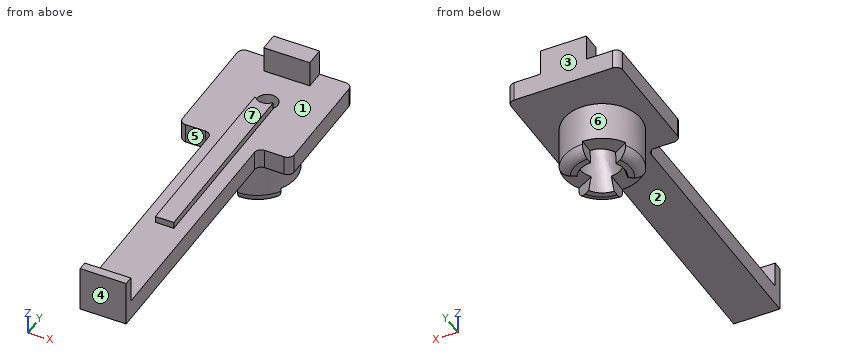
from build123d import *

# Parameters (mm, degrees)
SKETCH1_W           = 7
SKETCH1_H           = 56.5
BOSS_EXTRUDE1_DEPTH = 3
SKETCH2_W           = 2.8
SKETCH2_H           = 29
BOSS_EXTRUDE2_DEPTH = 1
SKETCH3_W           = 7
SKETCH3_H           = 2.85
SKETCH3_H_2         = 1.35
BOSS_EXTRUDE3_DEPTH = 4
SKETCH4_W           = 3
SKETCH4_H           = 18
BOSS_EXTRUDE4_DEPTH = 5
SKETCH5_W           = 3
SKETCH5_H           = 18
BOSS_EXTRUDE5_DEPTH = 5
SKETCH9_R           = 5.85
BOSS_EXTRUDE7_DEPTH = 8
FILLET1_R           = 1.5
FILLET2_R           = 1
SKETCH11_R          = 3.436863838
SKETCH7_R           = 1.6
CUT_EXTRUDE5_START  = -2
CUT_EXTRUDE5_DEPTH  = 2
SKETCH14_R          = 1.6
CUT_EXTRUDE6_DEPTH  = 3


with BuildPart() as part:
    # Sketch1 → Boss-Extrude1 (new body)
    with BuildSketch(Plane.XY):
        with Locations((0, 9.795104227)):
            Rectangle(SKETCH1_W, SKETCH1_H)
    extrude(amount=BOSS_EXTRUDE1_DEPTH)

    # Sketch2 → Boss-Extrude2 (add)
    with BuildSketch(Plane.XY.offset(3)):
        with Locations((0, 13.995104227)):
            Rectangle(SKETCH2_W, SKETCH2_H)
    extrude(amount=BOSS_EXTRUDE2_DEPTH)

    # Sketch3 → Boss-Extrude3 (add)
    with BuildSketch(Plane.XY.offset(3)):
        with Locations((0, 36.620104227)):
            Rectangle(SKETCH3_W, SKETCH3_H)
        with Locations((0, -17.779895773)):
            Rectangle(SKETCH3_W, SKETCH3_H_2)
    extrude(amount=BOSS_EXTRUDE3_DEPTH)

    # Sketch4 → Boss-Extrude4 (add)
    with BuildSketch(Plane.ZY.offset(3.5)):
        with Locations((1.5, 29.045104227)):
            Rectangle(SKETCH4_W, SKETCH4_H)
    extrude(amount=BOSS_EXTRUDE4_DEPTH)

    # Sketch5 → Boss-Extrude5 (add)
    with BuildSketch(Plane(origin=(3.5, 0, 0), x_dir=(0, 0, -1), z_dir=(1, 0, 0))):
        with Locations((-1.5, 29.045104227)):
            Rectangle(SKETCH5_W, SKETCH5_H)
    extrude(amount=BOSS_EXTRUDE5_DEPTH)

    # Sketch9 → Boss-Extrude7 (add)
    with BuildSketch(Plane(origin=(0, 0, 0), x_dir=(-1, 0, 0), z_dir=(0, 0, -1))):
        with Locations(Location((0, 26.670104227, 0), (0, 0, 180))):
            Circle(SKETCH9_R)
    extrude(amount=BOSS_EXTRUDE7_DEPTH)

    # Fillet1
    fillet1_edges = [part.edges().sort_by_distance(p)[0] for p in [
        (-5.85, 26.670104227, -8),
    ]]
    fillet(fillet1_edges, radius=FILLET1_R)

    # Fillet2
    fillet2_edges = [part.edges().sort_by_distance(p)[0] for p in [
        (-3.5, 20.045104227, 1.5),
        (-8.5, 20.045104227, 1.5),
        (-8.5, 38.045104227, 1.5),
        (3.5, 20.045104227, 1.5),
        (8.5, 38.045104227, 1.5),
        (8.5, 20.045104227, 1.5),
    ]]
    fillet(fillet2_edges, radius=FILLET2_R)

    # Sketch11 → Cut-Loft6 section 0
    with BuildSketch(Plane(origin=(0, 0, -8), x_dir=(-1, 0, 0), z_dir=(0, 0, -1))):
        with Locations((0, 26.670104227)):
            Circle(SKETCH11_R)
    # Sketch7 → Cut-Loft6 section 1
    with BuildSketch(Plane.XY.offset(3)):
        with Locations((0, 29.495104227)):
            Circle(SKETCH7_R)
    loft(mode=Mode.SUBTRACT)

    # Sketch10 → Cut-Extrude5 (cut)
    with BuildSketch(Plane(origin=(0, 0, -8), x_dir=(-1, 0, 0), z_dir=(0, 0, -1)).offset(CUT_EXTRUDE5_START)):
        with BuildLine():
            ThreePointArc((5.066248612, 29.595104227), (2.925, 31.736352839), (0, 32.520104227))
            Line((0, 32.520104227), (0, 26.670104227))
            Line((0, 26.670104227), (5.066248612, 29.595104227))
        make_face()
        with BuildLine():
            Line((5.066248612, 23.745104227), (0, 26.670104227))
            Line((0, 26.670104227), (0, 20.820104227))
            ThreePointArc((0, 20.820104227), (2.925, 21.603855615), (5.066248612, 23.745104227))
        make_face()
        with BuildLine():
            Line((-5.066248612, 23.745104227), (0, 26.670104227))
            Line((0, 26.670104227), (-5.066248612, 29.595104227))
            ThreePointArc((-5.066248612, 29.595104227), (-5.85, 26.670104227), (-5.066248612, 23.745104227))
        make_face()
    extrude(amount=CUT_EXTRUDE5_DEPTH, mode=Mode.SUBTRACT)

    # Sketch14 → Cut-Extrude6 (cut)
    with BuildSketch(Plane.XY.offset(3)):
        with Locations((0, 29.495104227)):
            Circle(SKETCH14_R)
    extrude(amount=CUT_EXTRUDE6_DEPTH, mode=Mode.SUBTRACT)


solid = part.part
Here's how the part is built. I have some questions about the finished solid (model axes, mm). Face numbers are marked on the shaded views. A direction names the side the tool comes from. Coordinates: 2 decimals unless noted, no trailing zeros. Order: outer loops, then holes, each group sorted by start corner. A loop starts at its lowest first (then second) coordinate and runs counter-clockwise, first axis right, second up.
Item 1: For P1, Ø1.5, axis at x = -6, z = 1, coming from the -Y side; P2, Ø5, axis at x = -4, y = -3, coming from the +Z side; P3, Ø2, axis at x = 0, y = 15, coming from the +Z side, each with a flat end and sliding along its axis, tell me the tip position at first contact or that it passes through.
Result sheet:
P1: stops at y = 20.05
P2: stops at z = 3
P3: stops at z = 4
Item 2: If we section it at B-B on y = 18: List the corners of the cut face in (x, z) for me, plus the area to 3 significant figures.
Result sheet:
outline: (-3.5, 0) - (3.5, 0) - (3.5, 3) - (1.4, 3) - (1.4, 4) - (-1.4, 4) - (-1.4, 3) - (-3.5, 3) - close
area: 23.8 mm2
Item 3: For the marked faces 4, 5, 6 and 7, which set-ups out of +Z, -Z, +X, -X, +Y, -Y let a thin tool reach every point of the face, with its end or its side?
Result sheet:
face 4: +Z, -Z, +X, -X, -Y
face 5: +Z, -Z, -X, -Y
face 6: -Z
face 7: +Z, +X, -X
Item 4: If we section it at A-A on z = 5.5: List the corners of the cut face in (x, y) for me, plus the area to 3 significant figures.
Result sheet:
outline: (-3.5, -18.45) - (3.5, -18.45) - (3.5, -17.1) - (-3.5, -17.1) - close; (-3.5, 35.2) - (3.5, 35.2) - (3.5, 38.05) - (-3.5, 38.05) - close
area: 29.4 mm2
Item 5: If we mould it in two halves opening along Y, with no side actions, what happens to the marked faces 1, 2 and 3? For each: +Y half, -Y half, draft (parallel to the pull), parting line (faces both ways), or undercut.
Result sheet:
face 1: undercut
face 2: draft
face 3: +Y half
Item 6: If we section it at C-C on y = -5: List the corners of the cut face in (x, z) for me, plus the area to 3 significant figures.
Result sheet:
outline: (-3.5, 0) - (3.5, 0) - (3.5, 3) - (-3.5, 3) - close
area: 21.0 mm2
Item 7: I need wall thicknesses on line 1 (Y direction, x = 0, z = 6); line 2 (Y direction, x = 6.25, z = 2.25); line 3 (Z direction, x = 3, y = 0.5). Which ranges of each line are inside material? Lowest first, please.
Result sheet:
line 1: y = -18.45 to -17.1, 35.2 to 38.05
line 2: y = 20.05 to 38.05
line 3: z = 0 to 3
